Design review of the part shown in the three views and the two pictorial views. Dimensions are in mm from the part's minimum x, y and z. Give positions to 0.01 mm unless a question says otherwise; leave off trailing zeros. Loops run counter-clockwise (first coordinate to the right, second up) from the corner with the lowest first, then second, coordinate; pieces in that order, holes last. Notation, with made-up numbers: M -6.5,22 L 49.5,22 A32 ccw 49.5,49 Z; hole C 42,-37 d1. An arc over 180 degrees is marked long. Return JSON: item names as keys, results as strings. Group by question number.
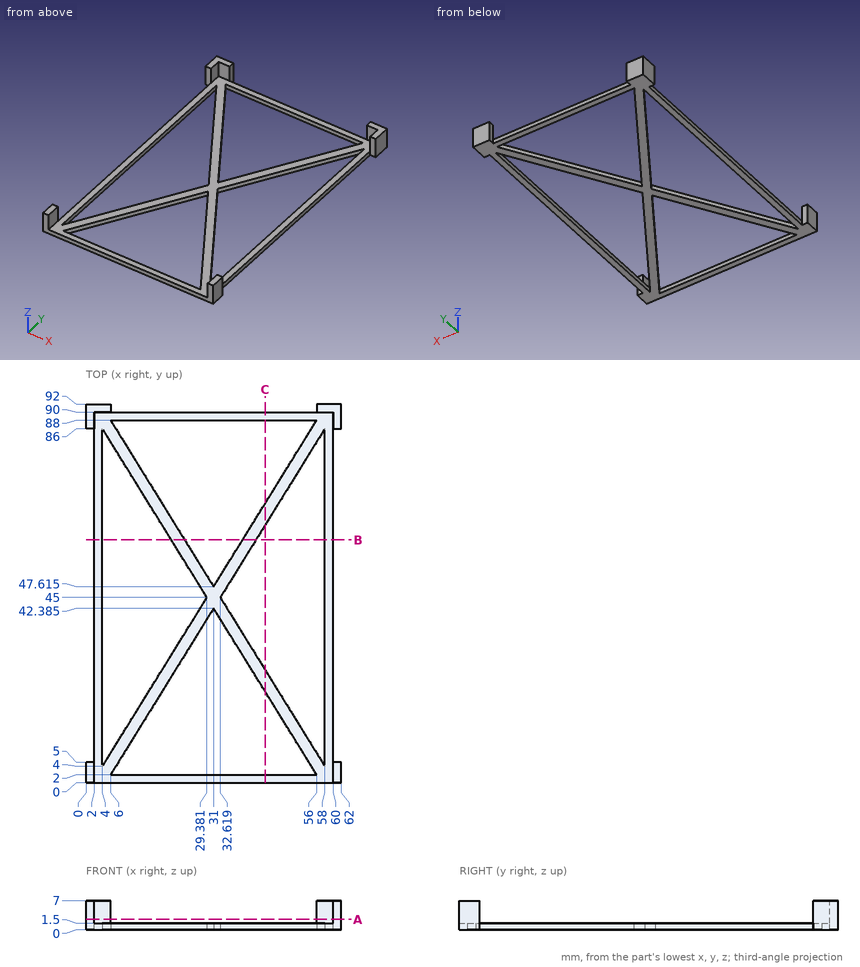
(1) Add section B-B (y = 59). Write out the cut boundary in (x, z) (1 decimal), and give its area (3 significant figures).
(2) For pin 1 (1.6 mm diameter, centred on x = 20, z = 1, fed in from +Y); pin 2 (2 mm diameter, centred on x = 4.5, z = 5.5, fed in from -Y); pin 3 (1 mm diameter, centred on x = 37, y = 51.5, fed in from +Z), all flat-tipped, find the tip position at first contact; note any pin that passes through.
(3) Add section A-A (z = 2.5). Write out the cut boundary in (x, y).
(4) For probe 1 along X at (y, z) = (45, 1); probe 2 along X at (y, z) = (6, 1.25) (1 decimal); probe 3 along Y at (x, z) = (44, 1) (1 decimal), list the stretches that pass through material, from the lowest coordinate up.
(5) Add section C-C (x = 43.5). Write out the cut boundary in (y, z), and give its area (3 significant figures).
Verdict:
{
 "1": {"outline": "M 2,0 L 4,0 L 4,1.5 L 2,1.5 Z; M 20.7,0 L 24,0 L 24,1.5 L 20.7,1.5 Z; M 38,0 L 41.3,0 L 41.3,1.5 L 38,1.5 Z; M 58,0 L 60,0 L 60,1.5 L 58,1.5 Z", "area": "15.7 mm²"},
 "2": {"pin 1": "stops at y = 90", "pin 2": "stops at y = 90", "pin 3": "stops at z = 1.5"},
 "3": {"outline": "M 0,0 L 2,0 L 2,5 L 0,5 Z; M 0,86 L 2,86 L 2,90 L 6,90 L 6,92 L 0,92 Z; M 56,90 L 60,90 L 60,86 L 62,86 L 62,92 L 56,92 Z; M 60,0 L 62,0 L 62,5 L 60,5 Z"},
 "4": {"probe 1": "x = 2 to 4, 29.38 to 32.62, 58 to 60", "probe 2": "x = 2 to 4, 5.2 to 8.5, 53.5 to 56.8, 58 to 60", "probe 3": "y = 0 to 2, 21.4 to 26.6, 63.4 to 68.6, 88 to 90"},
 "5": {"outline": "M 0,0 L 2,0 L 2,1.5 L 0,1.5 Z; M 22.19,0 L 27.42,0 L 27.42,1.5 L 22.19,1.5 Z; M 62.58,0 L 67.81,0 L 67.81,1.5 L 62.58,1.5 Z; M 88,0 L 90,0 L 90,1.5 L 88,1.5 Z", "area": "21.7 mm²"}
}
